from build123d import *

# Parameters (mm, degrees)
BOSS_EXTRUDE1_DEPTH           = 6.35
BOSS_EXTRUDE1_DEPTH_BACK      = 12.7
TAP_DRILL_FOR_6_32_TAP1_D     = 2.7051
TAP_DRILL_FOR_4_40_TAP1_D     = 2.2606
TAP_DRILL_FOR_4_40_TAP1_DEPTH = 3.302
TAP_DRILL_FOR_4_40_TAP1_TIP   = 0.679152758


with BuildPart() as part:
    # Sketch1 → Boss-Extrude1 (new body, two sides)
    with BuildSketch(Plane.XY) as boss_extrude1_sk:
        Polygon((-59.907074584, 30.83161157), (-40.857074584, 30.83161157), (-40.857074584, 5.43161157), (-44.032074584, 5.43161157), (-44.032074584, 27.65661157), (-59.907074584, 27.65661157), align=None)
    extrude(amount=BOSS_EXTRUDE1_DEPTH)
    extrude(boss_extrude1_sk.sketch, amount=-BOSS_EXTRUDE1_DEPTH_BACK)

    # Tap Drill for #6-32 Tap1 (through all)
    with Locations(Plane(origin=(-44.032074584, 11.78161157, 0), x_dir=(0, 0, -1), z_dir=(-1, 0, 0))):
        with Locations((0, 0), (6.35, -9.525)):
            Hole(TAP_DRILL_FOR_6_32_TAP1_D / 2)

    # Tap Drill for #4-40 Tap1
    with Locations(Plane(origin=(-51.458153967, 30.83161157, -7.531939217), x_dir=(0, 0, 1), z_dir=(0, 1, 0))):
        with Locations((0, 0), (7.531939217, -5.273920617)):
            Hole(TAP_DRILL_FOR_4_40_TAP1_D / 2, depth=TAP_DRILL_FOR_4_40_TAP1_DEPTH)
            with Locations((0, 0, -(TAP_DRILL_FOR_4_40_TAP1_DEPTH + TAP_DRILL_FOR_4_40_TAP1_TIP / 2))):  # 118° drill point
                Cone(0, TAP_DRILL_FOR_4_40_TAP1_D / 2, TAP_DRILL_FOR_4_40_TAP1_TIP, mode=Mode.SUBTRACT)


solid = part.part
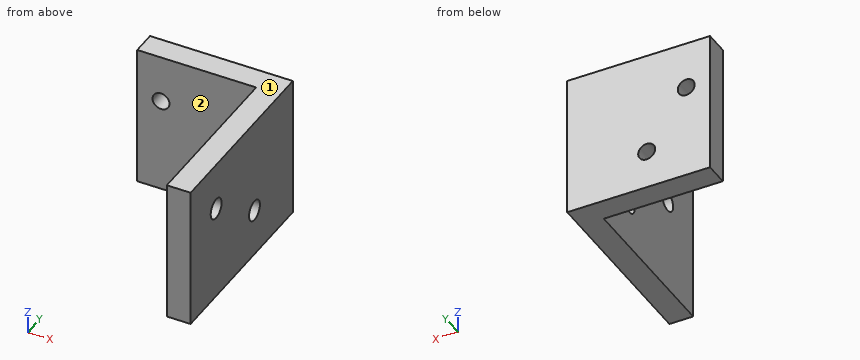
Design review of the part built by this model. Coordinates are the model's own, in mm. Face numbers are marked on the shaded views. A direction names the side the tool comes from. Give positions to 0.01 mm unless a question says otherwise; leave off trailing zeros. Loops run counter-clockwise (first coordinate to the right, second up) from the corner with the lowest first, then second, coordinate; pieces in that order, holes last. Notation, with made-up numbers: (-22, 38.5) - (0, 38.5) arc R15 ccw to (0, 64.5) - close; hole circle Ø5 at (13, 1.25). An arc over 180 degrees is marked (long way). Write item = value, one per line.
1) Take a section at D-D on z = -11.25. State the section outline as (x, y) points, and give its area (3 significant figures).
Result sheet:
outline = (-59.91, 27.66) - (-44.03, 27.66) - (-44.03, 5.43) - (-40.86, 5.43) - (-40.86, 30.83) - (-59.91, 30.83) - close
area = 131 mm2
2) Clearance check with flat-ended pins moving along their axes: pin 1 Ø5 at (y, z) = (11.5, 2) entering from -X; pin 2 Ø3 at (x, z) = (-56.73, 0) entering from -Y. State where each tip first meets the part, or that it passes through.
Result sheet:
pin_1 = -44.03
pin_2 = 27.66
3) To check wall thickness, follow line 1 (Y direction, x = -41.9, z = -6.35); line 2 (X direction, y = 15.5, z = -2.75); line 3 (Y direction, x = -47.75, z = -2.75). State the ranges of each line that lie inside material, in increasing order.
Result sheet:
line_1 = 5.43 to 19.95, 22.66 to 30.83
line_2 = -44.03 to -40.86
line_3 = 27.66 to 30.83
4) Tool access review of the marked faces 1 and 2: name each direction out of +Z, -Z, +X, -X, +Y, -Y from which nothing blocks a thin tool from reaching the whole face with its end or side.
Result sheet:
face_1 = +Z, +X, -X, +Y, -Y
face_2 = +Z, -Z, -X, -Y
5) Take a section at B-B on y = 20.5. State the section outline as (x, z) points.
Result sheet:
outline = (-44.03, -12.7) - (-40.86, -12.7) - (-40.86, -7.44) - (-44.03, -7.44) - close; (-44.03, -5.26) - (-40.86, -5.26) - (-40.86, 6.35) - (-44.03, 6.35) - close
6) Take a section at C-C on x = -57.25. State the section outline as (y, z) points, and give its area (3 significant figures).
Result sheet:
outline = (27.66, -12.7) - (30.83, -12.7) - (30.83, -1) - (27.66, -1) - close; (27.66, 1) - (30.83, 1) - (30.83, 6.35) - (27.66, 6.35) - close
area = 54.1 mm2
7) Take a section at A-A on z = 0. State the section outline as (x, y) points, and give its area (3 significant figures).
Result sheet:
outline = (-59.91, 27.66) - (-57.86, 27.66) - (-57.86, 30.83) - (-59.91, 30.83) - close; (-55.6, 27.66) - (-44.03, 27.66) - (-44.03, 13.13) - (-40.86, 13.13) - (-40.86, 30.83) - (-55.6, 30.83) - close; (-44.03, 5.43) - (-40.86, 5.43) - (-40.86, 10.43) - (-44.03, 10.43) - close
area = 115 mm2
